```python
from build123d import *

# Parameters (mm, degrees)
CROQUIS1_W              = 14.382940013
CROQUIS1_H              = 150
CROQUIS1_W_2            = 10
CROQUIS1_H_2            = 20
CROQUIS1_R              = 3.1
CROQUIS1_R_2            = 2.1
SALIENTE_EXTRUIR1_DEPTH = 2
CROQUIS2_W              = 14.382940013
CROQUIS2_H              = 150
CROQUIS2_R              = 4
SALIENTE_EXTRUIR2_DEPTH = 6
CROQUIS3_R              = 3.1
CORTAR_EXTRUIR1_DEPTH   = 4
CROQUIS4_R              = 2.1
CORTAR_EXTRUIR2_DEPTH   = 278.82310565
REDONDEO2_R             = 3


with BuildPart() as part:
    # Croquis1 → Saliente-Extruir1 (new body)
    # profile 1 of 3: a face of its own
    with BuildSketch(Plane(origin=(0, 0, -134.198862982), x_dir=(-1, 0, 0), z_dir=(0, 0, -1))):
        with Locations((-52.715326076, 163.447805519)):
            Rectangle(CROQUIS1_W, CROQUIS1_H)
        with Locations((-52.715326075, 163.447805519)):
            Rectangle(CROQUIS1_W_2, CROQUIS1_H_2, mode=Mode.SUBTRACT)
    # profile 2 of 3: a face of its own
    with BuildSketch(Plane(origin=(0, 0, -134.198862982), x_dir=(-1, 0, 0), z_dir=(0, 0, -1))):
        with Locations((-52.715326075, 163.447805519)):
            Rectangle(CROQUIS1_W_2, CROQUIS1_H_2)
        with Locations((-52.715326075, 163.447805519)):
            Circle(CROQUIS1_R, mode=Mode.SUBTRACT)
    # profile 3 of 3: a face of its own
    with BuildSketch(Plane(origin=(0, 0, -134.198862982), x_dir=(-1, 0, 0), z_dir=(0, 0, -1))):
        with Locations((-52.715326075, 163.447805519)):
            Circle(CROQUIS1_R)
        with Locations((-52.715326075, 163.447805519)):
            Circle(CROQUIS1_R_2, mode=Mode.SUBTRACT)
    extrude(amount=SALIENTE_EXTRUIR1_DEPTH)

    # Croquis2 → Saliente-Extruir2 (add)
    with BuildSketch(Plane(origin=(0, 0, -136.198862982), x_dir=(-1, 0, 0), z_dir=(0, 0, -1))):
        with Locations((-52.715326076, 163.447805519)):
            Rectangle(CROQUIS2_W, CROQUIS2_H)
        with Locations((-52.715326075, 163.447805519)):
            Circle(CROQUIS2_R, mode=Mode.SUBTRACT)
    extrude(amount=SALIENTE_EXTRUIR2_DEPTH)

    # Croquis3 → Cortar-Extruir1 (cut)
    with BuildSketch(Plane.ZY.offset(-45.523856069)):
        with Locations((-138.198862982, 93.447805519)):
            Circle(CROQUIS3_R)
        with Locations((-138.198862982, 233.447805519)):
            Circle(CROQUIS3_R)
    extrude(amount=-CORTAR_EXTRUIR1_DEPTH, mode=Mode.SUBTRACT)

    # Croquis4 → Cortar-Extruir2 (cut, through all)
    with BuildSketch(Plane.ZY.offset(-49.523856069)):
        with Locations((-138.198862982, 233.447805519)):
            Circle(CROQUIS4_R)
        with Locations((-138.198862982, 93.447805519)):
            Circle(CROQUIS4_R)
    extrude(amount=-CORTAR_EXTRUIR2_DEPTH, mode=Mode.SUBTRACT)

    # Redondeo2
    redondeo2_edges = [part.edges().sort_by_distance(p)[0] for p in [
        (52.715326075, 88.447805519, -142.198862982),
        (52.715326075, 238.447805519, -142.198862982),
        (52.715326075, 238.447805519, -134.198862982),
        (52.715326075, 88.447805519, -134.198862982),
    ]]
    fillet(redondeo2_edges, radius=REDONDEO2_R)


solid = part.part
```
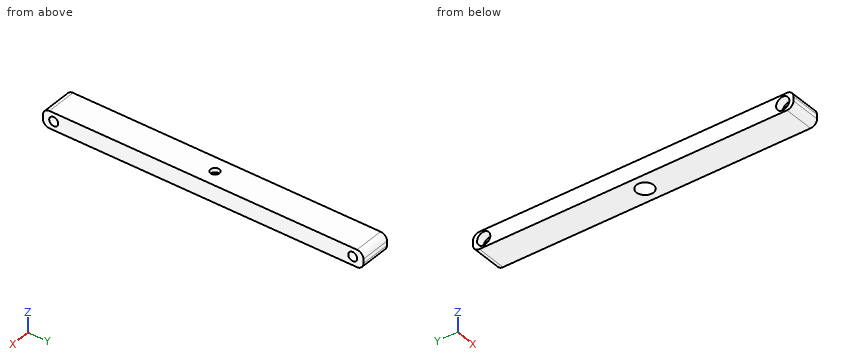
Design review of the part built by this model. Coordinates are the model's own, in mm. Give positions to 0.01 mm unless a question says otherwise; leave off trailing zeros. Loops run counter-clockwise (first coordinate to the right, second up) from the corner with the lowest first, then second, coordinate; pieces in that order, holes last. Notation, with made-up numbers: M -17,13 L 29,13 A27 ccw 29,49 Z; hole C 82.5,21 d8. An arc over 180 degrees is marked long. Return JSON: item names as keys, results as strings. Group by question number.
Item 1: We need section B-B (x = 58). Give the boundary of the cut face in (y, z).
Item 2: Insertion check: pin 1 Ø3 at (x, z) = (56.5, -135.5) entering from +Y; pin 2 Ø4 at (x, y) = (53, 164.5) entering from -Z; pin 3 Ø1.9 at (y, z) = (92, -139.5) entering from -X. Each pin has a flat end and moves straight along its axis. Give the tip position at first contact, or say it passes through.
Item 3: For probe 1 along Y at (x, z) = (51.5, -138.75); probe 2 along Y at (x, z) = (49.25, -136); probe 3 along Y at (x, z) = (55, -137), list the stretches that pass through material, from the lowest coordinate up.
Item 4: We need section A-A (x = 52). Give the boundary of the cut face in (y, z), and give its area (3 significant figures).
Output:
{
 "1": {"outline": "M 88.45,-139.2 A3 ccw 91.45,-142.2 L 235.45,-142.2 A3 ccw 238.45,-139.2 L 238.45,-137.2 A3 ccw 235.45,-134.2 L 91.45,-134.2 A3 ccw 88.45,-137.2 Z; hole C 93.45,-138.2 d4.2; hole C 233.45,-138.2 d4.2"},
 "2": {"pin 1": "stops at y = 238.44", "pin 2": "stops at z = -136.2", "pin 3": "stops at x = 49.52"},
 "3": {"probe 1": "y = 88.45 to 91.42, 95.47 to 159.64, 167.26 to 231.42, 235.47 to 238.45", "probe 2": "y = 88.7 to 91.26, 95.63 to 231.26, 235.63 to 238.2", "probe 3": "y = 88.45 to 91.72, 95.17 to 160.16, 166.73 to 231.72, 235.17 to 238.44"},
 "4": {"outline": "M 88.45,-139.2 A3 ccw 91.45,-142.2 L 159.51,-142.2 L 159.51,-136.2 L 161.47,-136.2 L 161.47,-134.2 L 91.45,-134.2 A3 ccw 88.45,-137.2 Z; M 165.42,-136.2 L 167.38,-136.2 L 167.38,-142.2 L 235.45,-142.2 A3 ccw 238.45,-139.2 L 238.45,-137.2 A3 ccw 235.45,-134.2 L 165.42,-134.2 Z; hole C 93.45,-138.2 d4.2; hole C 233.45,-138.2 d4.2", "area": "1,110 mm^2"}
}
